Verification items for the finished model (mm, model axes). A direction names the side the tool comes from. Coordinates: 2 decimals unless noted, no trailing zeros. Write each loop counter-clockwise with the first axis right and the second up, starting at its lowest first coordinate (ties: lowest second). Pieces come first, ordered by that corner, then holes. Notation, with made-up numbers: (1, 21.25) - (14, 21.25) arc R16 cw to (14, 52.25) - close; hole circle Ø2 at (21, -14). An arc over 180 degrees is marked (long way). Use one line per item in the form item = value. Start each with the question number.
(1) Tool access check on faces 1 (the cylindrical face through (41.52, 10.98, 2.54)), 2 (the flat face through (41.994, 4, 3)), 3 (the flat face through (34.98, 18.36, 3.03)), 4 (the cylindrical face through (5.463, 10.896, 2.535)). Record the directions out of +Z, -Z, +X, -X, +Y, -Y that give a thin tool (end or side, any length) a straight path to the whole face; none if there is none.
(2) Sectioned sample at A-A (z = 7.5). Record the cut outline in (x, y).
(3) Sectioned sample at B-B (y = 10.25). Record the cut outline in (x, z), and give its area (3 significant figures).
(4) Material ranges on line 1 (X direction, y = 3.5, z = 5.5); line 2 (X direction, y = 14.5, z = 2); line 3 (Y direction, x = 13.5, z = 3.5), recorded low to high. Write a range as [from, to].
(5) Sectioned sample at C-C (x = 10). Record the cut outline in (y, z).
(6) Mould release check, pull along Y, two halves, no side actions. Record for faces 5 (the cylindrical face through (6.096, 7.008, 3.028)), 6 (the flat face through (5.014, 4, 3)), 7 (the cylindrical face through (32.94, 27.1, 2.54)): released by +Y, released by -Y, zero draft, split by the parting line, or undercut.
(7) Sectioned sample at D-D (z = 2.75). Record the cut outline in (x, y).
(8) Gauge pin test, flat ends, axial feed: pin 1 Ø1.8 at (y, z) = (4, 2) entering from +X; pin 2 Ø3 at (y, z) = (5, 2) entering from -X; pin 3 Ø1.5 at (x, y) = (37, 19.5) entering from -Z; pin 4 Ø1.5 at (x, z) = (30, 2.5) entering from -Y. Record the tip position at first contact, or that the pin passes through.
from build123d import *

# Parameters (mm, degrees)
SKETCH_1_W               = 47
SKETCH_1_H               = 32
EXTRUDE_1_DEPTH          = 5
CUT_EXTRUDE_1_DEPTH      = 58.078892771
CUT_EXTRUDE_5_DEPTH      = 4
CUT_EXTRUDE_6_DEPTH      = 58.078892771
SKETCH_5_W               = 0.757642216
SKETCH_5_H               = 6
SKETCH_5_W_2             = 0.766357784
EXTRUDE_2_DEPTH          = 5
CUT_EXTRUDE_7_DEPTH      = 54.728894948
CUT_EXTRUDE_8_DEPTH      = 55.418489547
SKETCH_8_W               = 47
SKETCH_8_H               = 2
CUT_EXTRUDE_9_DEPTH      = 10
CUT_EXTRUDE_START        = -0.814789408
CUT_EXTRUDE_10_OUTLINE_W = 4.001231447
CUT_EXTRUDE_10_OUTLINE_H = 5
CUT_EXTRUDE_10_DEPTH     = 0.814789408


# Read off the part's stored shape, not the designer's step: 切除-拉伸10
with BuildPart() as part:
    # 草图1 → 凸台-拉伸1 (new body)
    with BuildSketch(Plane.XY):
        with Locations((23.5, 16)):
            Rectangle(SKETCH_1_W, SKETCH_1_H)
    extrude(amount=EXTRUDE_1_DEPTH)

    # 草图2 → 切除-拉伸1 (cut, through all)
    with BuildSketch(Plane.XY.offset(5)):
        with BuildLine():
            Line((23.5, 0), (23.5, 26))
            Line((23.5, 26), (18.566996488, 26))
            ThreePointArc((18.566996488, 26), (18.15387041, 25.873934732), (17.881511675, 25.538694031))
            Line((17.881511675, 25.538694031), (7.626711155, 0.31171158))
            ThreePointArc((7.626711155, 0.31171158), (7.442674144, 0.085184252), (7.163518462, 0))
            Line((7.163518462, 0), (7.5, 0))
            Line((7.5, 0), (23.5, 0))
        make_face()
        with BuildLine():
            Line((28.45115486, 26), (23.5, 26))
            Line((23.5, 26), (23.5, 0))
            Line((23.5, 0), (39.5, 0))
            Line((39.5, 0), (39.836703186, 0))
            ThreePointArc((39.836703186, 0), (39.557420976, 0.085269428), (39.373395704, 0.311994211))
            Line((39.373395704, 0.311994211), (29.136809551, 25.538275761))
            ThreePointArc((29.136809551, 25.538275761), (28.864468188, 25.873808678), (28.45115486, 26))
        make_face()
    extrude(amount=-CUT_EXTRUDE_1_DEPTH, mode=Mode.SUBTRACT)

    # 草图3 → 切除-拉伸5 (cut)
    with BuildSketch(Plane.XY.offset(5)):
        with BuildLine():
            Line((28.45115486, 26), (18.566996488, 26))
            add(Edge.make_bspline(
                [(18.566996488, 26), (18.083486738, 25.978522449), (17.881511675, 25.538694031)],
                knots=[0, 0, 0, 1, 1, 1], degree=2))
            Line((17.881511675, 25.538694031), (7.614040039, 0.280540422))
            ThreePointArc((7.614040039, 0.280540422), (7.448406729, 0.076665827), (7.197166615, 0))
            Line((7.197166615, 0), (5.772, 0))
            Line((5.772, 0), (5.772, 4.436119664))
            ThreePointArc((5.772, 4.436119664), (6.104843669, 7.043618399), (7.082028835, 9.483893735))
            Line((7.082028835, 9.483893735), (16.830389156, 27))
            Line((16.830389156, 27), (30.169610844, 27))
            Line((30.169610844, 27), (39.917971165, 9.483893735))
            ThreePointArc((39.917971165, 9.483893735), (40.895156331, 7.043618399), (41.228, 4.436119664))
            Line((41.228, 4.436119664), (41.228, 0))
            Line((41.228, 0), (39.803032868, 0))
            ThreePointArc((39.803032868, 0), (39.551678879, 0.076742485), (39.386056133, 0.28079479))
            Line((39.386056133, 0.28079479), (29.136809551, 25.538275761))
            add(Edge.make_bspline(
                [(28.45115486, 26), (28.93495417, 25.978479476), (29.136809551, 25.538275761)],
                knots=[0, 0, 0, 1, 1, 1], degree=2))
        make_face()
    extrude(amount=-CUT_EXTRUDE_5_DEPTH, mode=Mode.SUBTRACT)

    # 草图4 → 切除-拉伸6 (cut, through all)
    with BuildSketch(Plane.XY.offset(5)):
        with BuildLine():
            Line((0, 0), (5.014357784, 0))
            Line((5.014357784, 0), (5.014357784, 7.877425761))
            ThreePointArc((5.014357784, 7.877425761), (5.475718856, 10.937654809), (6.818789734, 13.72584714))
            Line((6.818789734, 13.72584714), (14.045555305, 24.365213617))
            ThreePointArc((14.045555305, 24.365213617), (13.978253194, 27.216535436), (11.556446219, 28.722993754))
            Line((11.556446219, 28.722993754), (0, 29.43))
            Line((0, 29.43), (0, 0))
        make_face()
        with BuildLine():
            Line((41.994357784, 7.873314412), (41.994357784, 0))
            Line((41.994357784, 0), (47, 0))
            Line((47, 0), (47, 29.43))
            Line((47, 29.43), (35.433873083, 28.73462187))
            ThreePointArc((35.433873083, 28.73462187), (32.920113477, 27.060422918), (33.13664909, 24.047941912))
            Line((33.13664909, 24.047941912), (40.185693822, 13.727936391))
            ThreePointArc((40.185693822, 13.727936391), (41.531889434, 10.937130001), (41.994357784, 7.873314412))
        make_face()
    extrude(amount=-CUT_EXTRUDE_6_DEPTH, mode=Mode.SUBTRACT)

    # 草图5 → 凸台-拉伸2 (add)
    with BuildSketch(Plane.XY.offset(5)):
        with Locations((5.393178892, 3)):
            Rectangle(SKETCH_5_W, SKETCH_5_H)
        with Locations((41.611178892, 3)):
            Rectangle(SKETCH_5_W_2, SKETCH_5_H)
    extrude(amount=EXTRUDE_2_DEPTH)

    # 草图6 → 切除-拉伸7 (cut, through all)
    with BuildSketch(Plane.ZY.offset(-5.014357784)):
        Polygon((6.053573934, 5.25247322), (10, 4.6), (10, 6), (5, 6), align=None)
        Polygon((10, 0), (10, 1.4), (6.053573934, 0.757008468), (5, 0), align=None)
    extrude(amount=-CUT_EXTRUDE_7_DEPTH, mode=Mode.SUBTRACT)

    # 草图7 → 切除-拉伸8 (cut, through all)
    with BuildSketch(Plane(origin=(0, 6.086940952, 1.006370294), x_dir=(1, 0, 0), z_dir=(0, 0.9866065166041178, 0.16311830490257262))):
        Polygon((5.1771781, -9.637699539), (5.158383514, -9.115720963), (5.014357784, -9.115720963), (5.014357784, -9.637699539), align=None)
        Polygon((5.158383514, -9.115720963), (5.014357784, -5.115720963), (5.014357784, -9.115720963), align=None)
        Polygon((5.772, -9.115720963), (5.772, -5.115720963), (5.627806352, -9.115720963), align=None)
        Polygon((5.772, -9.115720963), (5.627806352, -9.115720963), (5.608989853, -9.637699539), (5.772, -9.637699539), align=None)
        Polygon((41.994357784, -9.637699539), (41.994357784, -5.115720963), (41.862646969, -9.637699539), align=None)
        Polygon((41.390820316, -9.637699539), (41.228, -5.115720963), (41.228, -9.637699539), align=None)
    extrude(amount=-CUT_EXTRUDE_8_DEPTH, mode=Mode.SUBTRACT)

    # 草图8 → 切除-拉伸9 (cut)
    with BuildSketch(Plane.XY.offset(5)):
        with Locations((23.5, 31)):
            Rectangle(SKETCH_8_W, SKETCH_8_H)
    extrude(amount=-CUT_EXTRUDE_9_DEPTH, mode=Mode.SUBTRACT)

    # 切除-拉伸10 outline → 切除-拉伸10 (cut)
    with BuildSketch(Plane(origin=(0, 30, 0), x_dir=(1, 0, 0), z_dir=(0, 1, 0)).offset(CUT_EXTRUDE_START)):
        with Locations((2.000615724, -2.5)):
            Rectangle(CUT_EXTRUDE_10_OUTLINE_W, CUT_EXTRUDE_10_OUTLINE_H)
        with Locations((44.999384277, -2.5)):
            Rectangle(CUT_EXTRUDE_10_OUTLINE_W, CUT_EXTRUDE_10_OUTLINE_H)
    extrude(amount=CUT_EXTRUDE_10_DEPTH, mode=Mode.SUBTRACT)


solid = part.part
Answers below:
q1.face_1 = +Z, -Z, +X
q1.face_2 = +Z, -Z, +X, -Y
q1.face_3 = +Z, -Y
q1.face_4 = +Z, -Z, -X
q2.outline = (5.07, 5.01) - (5.09, 0.99) - (5.7, 0.99) - (5.72, 5.01) - close; (41.28, 5.01) - (41.3, 0.99) - (41.93, 0.99) - (41.95, 5.01) - close
q3.outline = (5.29, 0) - (11.67, 0) - (11.67, 1) - (7.51, 1) - (7.51, 5) - (5.29, 5) - close; (35.34, 0) - (41.72, 0) - (41.72, 5) - (39.49, 5) - (39.49, 1) - (35.34, 1) - close
q3.area = 30.5 mm2
q4.line_1 = [5.01, 5.77], [41.23, 41.99]
q4.line_2 = [7.34, 9.87], [37.13, 39.66]
q4.line_3 = [21.02, 23.56], [27.84, 30]
q5.outline = (6.15, 0) - (18.41, 0) - (18.41, 5) - (14.73, 5) - (14.73, 1) - (6.15, 1) - close; (28.82, 0) - (30, 0) - (30, 5) - (28.82, 5) - close
q6.face_5 = released by -Y
q6.face_6 = zero draft
q6.face_7 = undercut
q7.outline = (4, 29.19) - (11.56, 28.72) arc R3 cw to (14.05, 24.37) - (6.82, 13.73) arc R10.38 ccw to (5.01, 7.88) - (5.01, 0) - (5.77, 0) - (5.77, 4.44) arc R10.38 cw to (7.08, 9.48) - (16.83, 27) - (30.17, 27) - (39.92, 9.48) arc R10.38 cw to (41.23, 4.44) - (41.23, 0) - (41.99, 0) - (41.99, 7.87) arc R10.38 ccw to (40.19, 13.73) - (33.14, 24.05) arc R3 cw to (35.43, 28.73) - (43, 29.19) - (43, 30) - (4, 30) - close
q8.pin_1 = 41.99
q8.pin_2 = 5.01
q8.pin_3 = 0
q8.pin_4 = 25.96
